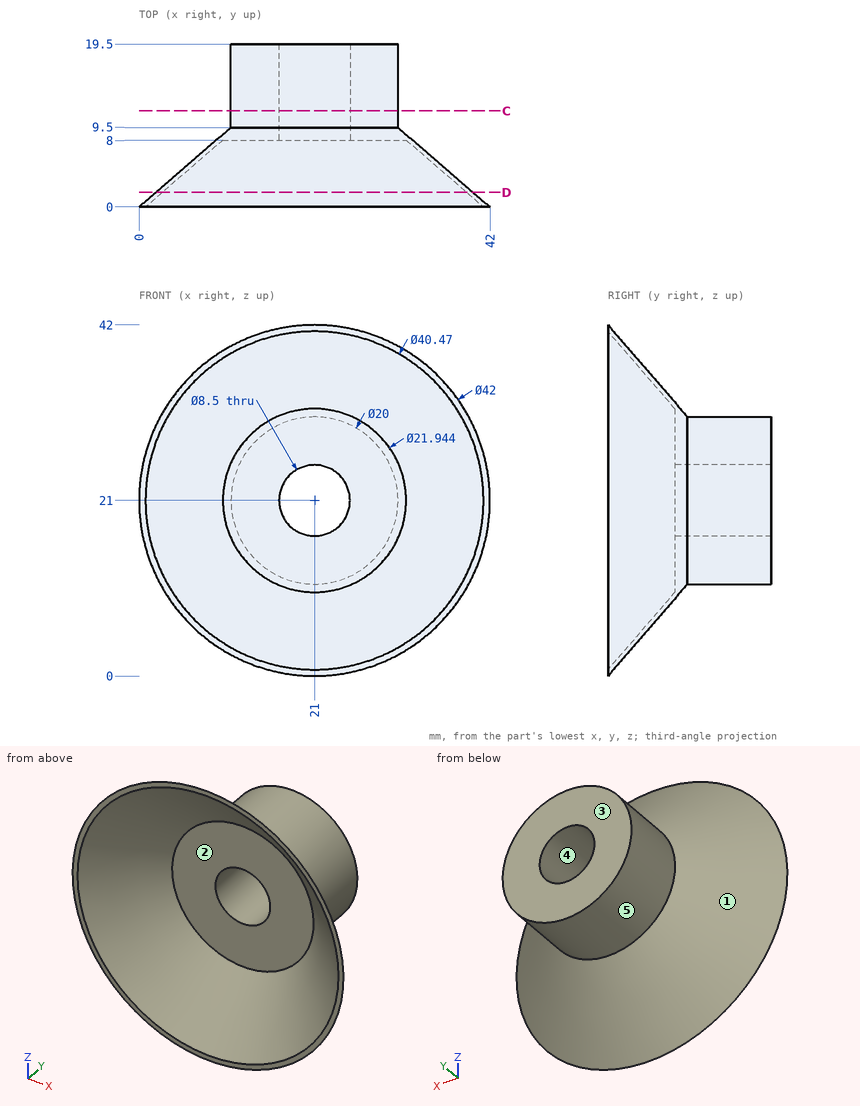
Answer from the drawing. Dimensions are ordinates in mm from the lowest x, y and z of the part. A direction names the side the tool comes from. Round coordinates to 2 decimals unless told otherwise and drop trailing zeros. Write each loop counter-clockwise with the first axis right and the second up, starting at its lowest first coordinate (ties: lowest second). Pieces come first, ordered by that corner, then holes. Notation, with made-up numbers: M 58.5,49 L 89.5,49 A17 cw 89.5,70 Z; hole C 68,88 d10. An arc over 180 degrees is marked long. One line per item, written item: value.
Q1. Straight lines are drawn through the part: line 1 (Z direction, x = 21, y = 15.25); line 2 (X direction, y = 6.5, z = 14.5). For each, find the intervals that lie inside material, in ascending order. Write a range as [from, to].
Data:
line 1: [11, 16.75], [25.25, 31]
line 2: [9.2, 10.08], [31.92, 32.8]
Q2. For a pull along Z with two mould halves and no side action, classify the marked faces 3, 4 and 5 as +Z half, -Z half, draft (parallel to the pull), parting line (faces both ways), or undercut.
Data:
face 3: draft
face 4: undercut
face 5: parting line
Q3. Which of the six approach directions +Z, -Z, +X, -X, +Y, -Y give full straight-line access (tool end or side, diameter ignored) to the marked faces 1 and 2?
Data:
face 1: +Y
face 2: -Y
Q4. Flat-ended cylindrical pins translate along their axes: pin 1 Ø7.5 at (x, z) = (21, 21) entering from +Y; pin 2 Ø17.5 at (x, z) = (20, 19.5) entering from -Y; pin 3 Ø2 at (y, z) = (8.5, 12) entering from -X; pin 4 Ø10 at (x, z) = (21.5, 5) entering from +Y. Find the tip coordinate at first contact, or state that the pin passes through.
Data:
pin 1: through
pin 2: y = 8
pin 3: x = 12.3
pin 4: y = 8.63
Q5. Find section C-C on y = 11.5. Write down the section's boundary in (x, z).
Data:
outline: C 21,21 d20; hole C 21,21 d8.5
Q6. Find section D-D on y = 1.75. Write down the section's boundary in (x, z).
Data:
outline: C 21,21 d37.95; hole C 21,21 d36.42
